Autodesk Inventor part; units mm, degrees
ref_plane "YZ Plane" through (0, 0, 0) normal (1, 0, 0) x (0, 1, 0)
ref_plane "XZ Plane" through (0, 0, 0) normal (0, 1, 0) x (-1, 0, 0)
ref_plane "XY Plane" through (0, 0, 0) normal (0, 0, 1) x (1, 0, 0)
sketch "Sketch1" plane through (0, 0, 0) normal (0, 0, 1) x (1, 0, 0)
  circle A0 centre (0, 0) radius 6
  line L0 (-3, -5.1962) -> (-7.3323, -12.7)
  line L1 (-7.3323, -12.7) -> (7.3323, -12.7)
  line L2 (7.3323, -12.7) -> (3, -5.1962)
  line L3 (-7.5, -22.5) -> (7.5, -22.5)
  line L4 (7.5, -22.5) -> (7.5, -12.7)
  line L5 (7.5, -12.7) -> (-7.5, -12.7)
  line L6 (-7.5, -12.7) -> (-7.5, -22.5)
  line L7 (0, -12.7) -> (0, 0)
  line L8 (-15, -18) -> (15, -18)
  line L9 (15, -18) -> (15, -22.5)
  line L10 (15, -22.5) -> (-15, -22.5)
  line L11 (-15, -22.5) -> (-15, -18)
  point P0 (0, -22.5)
  dimension "d0" = 12
  dimension "d1" = 60
  dimension "d2" = 3
  dimension "d3" = 3
  dimension "d4" = 15
  dimension "d5" = 9.8
  dimension "d7" = 4.5
  dimension "d8" = 30
  dimension "d31" = 22.5
extrude "Extrusion1" add sketch "Sketch1" along normal blind 350
sketch "Sketch2" plane through (0, 0, 350) normal (0, 0, 1) x (1, 0, 0)
  arc A0 (3, -5.1962) -> (-3, -5.1962) centre (0, 0) ccw
  line L0 (3, -5.1962) -> (7.3323, -12.7)
  line L1 (7.3323, -12.7) -> (7.5, -12.7)
  line L2 (7.5, -12.7) -> (7.5, -18)
  line L3 (7.5, -18) -> (15, -18)
  line L4 (15, -18) -> (15, -22.5)
  line L5 (15, -22.5) -> (-15, -22.5)
  line L6 (-15, -22.5) -> (-15, -18)
  line L7 (-15, -18) -> (-7.5, -18)
  line L8 (-7.5, -18) -> (-7.5, -12.7)
  line L9 (-7.5, -12.7) -> (-7.3323, -12.7)
  line L10 (-7.3323, -12.7) -> (-3, -5.1962)
  line L11 (-6, -21.5) -> (6, -21.5)
  line L12 (6, -21.5) -> (6, -22.5)
  line L13 (6, -22.5) -> (-6, -22.5)
  line L14 (-6, -22.5) -> (-6, -21.5)
  point P0 (0, -22.5)
  dimension "d11" = 12
  dimension "d12" = 1
extrude "Extrusion2" cut sketch "Sketch2" against normal through all contours L5 L14 L11 L12
chamfer "Chamfer1" distance 1 angle 45 2 edges at (-6, -21.5, 175) (6, -21.5, 175)
sketch "Sketch3" plane through (-15, -22.5, 0) normal (0, -1, 0) x (1, 0, 0)
  line L0 (21, 0) -> (21, 350) construction
  line L1 (21, 350) -> (30, 350)
  line L2 (30, 350) -> (30, 0)
  line L3 (30, 0) -> (21, 0) construction
  line L4 (9, 350) -> (9, 0) construction
  line L5 (9, 0) -> (0, 0) construction
  line L6 (0, 0) -> (0, 350)
  line L7 (0, 350) -> (9, 350)
  circle A0 centre (4, 25) radius 2
  circle A1 centre (26, 25) radius 2
  line L8 (26, 25) -> (4, 25) construction
  line L9 (15, 25) -> (15, 0) construction
  dimension "d18" = 25
  dimension "d19" = 4
  dimension "d20" = 4
  dimension "d21" = 22
extrude "Extrusion3" cut sketch "Sketch3" against normal through all
thread "Thread1"
thread "Thread2"
pattern_linear "Rectangular Pattern1" count 4 spacing 100 along (0, 0, 1) of "Extrusion3"
properties part number "sbr12_350mm"
Geometry: final body of the model. Coordinates: model frame, mm. A direction names the side the tool comes from. Round coordinates to 2 decimals unless told otherwise and drop trailing zeros. Order: outer loops, then holes, each group sorted by start corner. A loop starts at its lowest first (then second) coordinate and runs counter-clockwise, first axis right, second up. Notation, with made-up numbers: M 62,88.5 L 66,88.5 A8 ccw 66,99.5 Z; hole C 51,57.25 d5. An arc over 180 degrees is marked long. Use one line per item in the form item = value. Start each with the question number.
Q1. Pin query (flat end, axial travel): pin 1 Ø6 at (x, y) = (-7, -18.5) entering from -Z; pin 2 Ø3 at (x, z) = (11, 325) entering from -Y; pin 3 Ø5 at (x, z) = (11, 125) entering from +Y; pin 4 Ø12 at (x, z) = (-10.5, 72) entering from +Y. Return the tip coordinate at first contact, or that it passes through.
Q2. Access query for faces 4 (the face through (-11, -18, 173)), 5 (the face through (0, -21.5, 177)), 6 (the face through (7.5, -15, 173)), 7 (the face through (5.196, -9.001, 172.55)), 8 (the face through (-5.14, -8.9, 172.55)). Directions: +Z, -Z, +X, -X, +Y, -Y. A direction counts if a zero-diameter tool reaches every point of the face in a straight line with its end or side. Return the directions, or none.
Q3. Mould query, pull axis Y, two halves, no side actions, for faces 1 (the face through (11, -18, 173)), 2 (the face through (0, -11, 350)), 3 (the face through (0, 6, 173)). Classes: +Y half, -Y half, draft (parallel to the pull), parting line (faces both ways), or undercut.
Q4. Cut plane A-A (y = 0). Return loops of the section in (x, z).
Q5. Material intervals for line 1 (Z direction, x = 11, y = -21); line 2 (X direction, y = -20, z = 225); line 3 (Y direction, x = -9, z = 168), sorted ascending. Write a range as [from, to].
Geometry results:
q1.pin_1 = 0
q1.pin_2 = through
q1.pin_3 = -18
q1.pin_4 = 3.97
q2.face_4 = +Z, -Z, -X, +Y
q2.face_5 = +Z, -Z, -Y
q2.face_6 = +Z, -Z, +X, +Y
q2.face_7 = +Z, -Z, +X
q2.face_8 = +Z, -Z, -X
q3.face_1 = +Y half
q3.face_2 = draft
q3.face_3 = undercut
q4.outline = M -6,0 L 6,0 L 6,350 L -6,350 Z
q5.line_1 = [0, 23], [27, 123], [127, 223], [227, 323], [327, 350]
q5.line_2 = [-15, -13], [-9, 9], [13, 15]
q5.line_3 = [-22.5, -18]
